```python
from build123d import *

# Parameters (mm, degrees)
SKETCH1_W                  = 15
SKETCH1_H                  = 20
BOSS_EXTRUDE1_DEPTH        = 10
F_4_2_4_2_DIAMETER_HOLE1_D = 4.2
SKETCH4_W                  = 10
SKETCH4_H                  = 20
BOSS_EXTRUDE2_DEPTH        = 15
SKETCH5_W                  = 15
SKETCH5_H                  = 20
BOSS_EXTRUDE3_DEPTH        = 20
CHAMFER1_SIZE              = 10
CHAMFER2_SIZE              = 15
SKETCH6_W                  = 5
SKETCH6_H                  = 20
CUT_EXTRUDE1_DEPTH         = 10
SKETCH8_W                  = 15
SKETCH8_H                  = 20
BOSS_EXTRUDE4_DEPTH        = 10
CHAMFER3_SIZE              = 10
SKETCH7_W                  = 10
SKETCH7_H                  = 20
BOSS_EXTRUDE5_DEPTH        = 25
FILLET5_R                  = 3.175
SKETCH9_W                  = 10
SKETCH9_H                  = 10
CUT_EXTRUDE4_DEPTH         = 37
SKETCH15_W                 = 35.287710309
SKETCH15_H                 = 35.27052657
CUT_EXTRUDE5_DEPTH         = 10
SKETCH16_W                 = 32
SKETCH16_H                 = 10
CUT_EXTRUDE6_DEPTH         = 46
MOVE_FACE1_BY              = 5
SKETCH19_W                 = 2
SKETCH19_H                 = 6.2
BOSS_EXTRUDE6_DEPTH        = 2
FILLET6_R                  = 6.35
FILLET7_R                  = 3.175


# Some blends are built 0.0001 mm under size
with BuildPart() as part:
    # Sketch1 → Boss-Extrude1 (new body)
    with BuildSketch(Plane.XY):
        with Locations((7.5, 10)):
            Rectangle(SKETCH1_W, SKETCH1_H)
    extrude(amount=BOSS_EXTRUDE1_DEPTH)

    # Ø4.2 (4.2) Diameter Hole1 (through all)
    with Locations(Plane.XY.offset(10)):
        with Locations((8, 17)):
            Hole(F_4_2_4_2_DIAMETER_HOLE1_D / 2)

    # Sketch4 → Boss-Extrude2 (add)
    with BuildSketch(Plane(origin=(15, 0, 0), x_dir=(0, 0, -1), z_dir=(1, 0, 0))):
        with Locations((-5, 10)):
            Rectangle(SKETCH4_W, SKETCH4_H)
    extrude(amount=BOSS_EXTRUDE2_DEPTH)

    # Sketch5 → Boss-Extrude3 (add)
    with BuildSketch(Plane(origin=(0, 0, 0), x_dir=(-1, 0, 0), z_dir=(0, 0, -1))):
        with Locations((-22.5, 10)):
            Rectangle(SKETCH5_W, SKETCH5_H)
    extrude(amount=BOSS_EXTRUDE3_DEPTH)

    # Chamfer1
    # the kernel refuses this chamfer: 10 mm, written as the material it adds along each edge
    with BuildSketch(Plane(origin=(15, 20, 0), x_dir=(-0.9996219169112968, 0, 0.027495876610586372), z_dir=(0, -1, 0))) as chamfer1_piece_1_section:
        Polygon((CHAMFER1_SIZE * 0.999621916911, CHAMFER1_SIZE * 0.0274958766106), (-CHAMFER1_SIZE * 0.0274958766106, CHAMFER1_SIZE * 0.999621916911), (0, 0), align=None)
    chamfer1_piece_1 = extrude(amount=20, mode=Mode.PRIVATE)
    chamfer1_piece_1 = chamfer1_piece_1 - Plane(origin=(8, 17, -3.373966189), x_dir=(-1, 0, 0), z_dir=(0, 0, -1)) * Cylinder(2.1, 80, mode=Mode.PRIVATE)
    add(chamfer1_piece_1)

    # Chamfer2
    chamfer2_edges = [part.edges().sort_by_distance(p)[0] for p in [
        (30, 10, 10),
    ]]
    chamfer(chamfer2_edges, length=CHAMFER2_SIZE)

    # Sketch6 → Cut-Extrude1 (cut)
    with BuildSketch(Plane(origin=(0, 0, 0), x_dir=(-1, 0, 0), z_dir=(0, 0, -1))):
        with Locations((-2.5, 10)):
            Rectangle(SKETCH6_W, SKETCH6_H)
    extrude(amount=-CUT_EXTRUDE1_DEPTH, mode=Mode.SUBTRACT)

    # Sketch8 → Boss-Extrude4 (add)
    with BuildSketch(Plane(origin=(30, 0, 0), x_dir=(0, 0, -1), z_dir=(1, 0, 0))):
        with Locations((12.5, 10)):
            Rectangle(SKETCH8_W, SKETCH8_H)
    extrude(amount=BOSS_EXTRUDE4_DEPTH)

    # Chamfer3
    chamfer3_edges = [part.edges().sort_by_distance(p)[0] for p in [
        (40, 10, -5),
    ]]
    chamfer(chamfer3_edges, length=CHAMFER3_SIZE - 0.0001)  # a hair under: the kernel refuses the full size

    # Sketch7 → Boss-Extrude5 (add)
    with BuildSketch(Plane(origin=(30, 0, 0), x_dir=(0, 0, -1), z_dir=(1, 0, 0))):
        with Locations((15, 10)):
            Rectangle(SKETCH7_W, SKETCH7_H)
    extrude(amount=BOSS_EXTRUDE5_DEPTH)

    # Fillet5
    fillet5_edges = [part.edges().sort_by_distance(p)[0] for p in [
        (35.0001, 10, -10),
    ]]
    fillet(fillet5_edges, radius=FILLET5_R)

    # Sketch9 → Cut-Extrude4 (cut)
    with BuildSketch(Plane(origin=(0, 0, -20), x_dir=(-1, 0, 0), z_dir=(0, 0, -1))):
        with Locations((-10, 5)):
            Rectangle(SKETCH9_W, SKETCH9_H)
    extrude(amount=-CUT_EXTRUDE4_DEPTH, mode=Mode.SUBTRACT)

    # Sketch14 → CBORE for M5 SBHCS2 (revolve, cut)
    with BuildSketch(Plane(origin=(45, 10, 10), x_dir=(0, -1, 0), z_dir=(1, 0, 0))):
        Polygon((0, 0), (0, 30), (2.65, 30), (2.65, 22.75), (5.25, 22.75), (5.25, 0.020977491), (5.275, 0), align=None)
    revolve(axis=Axis((45, 10, 16.35), (0, 0, -1)), mode=Mode.SUBTRACT)

    # Sketch15 → Cut-Extrude5 (cut)
    with BuildSketch(Plane(origin=(2.5, 0, 2.5), x_dir=(-0.707106781186544, 0, 0.7071067811865511), z_dir=(-0.7071067811865511, 0, -0.707106781186544))):
        with Locations((-14.684853065, 9.385409348)):
            Rectangle(SKETCH15_W, SKETCH15_H)
    extrude(amount=CUT_EXTRUDE5_DEPTH, mode=Mode.SUBTRACT)

    # Sketch16 → Cut-Extrude6 (cut)
    with BuildSketch(Plane(origin=(0, 0, -20), x_dir=(-1, 0, 0), z_dir=(0, 0, -1))):
        with Locations((-21, 5)):
            Rectangle(SKETCH16_W, SKETCH16_H)
    extrude(amount=-CUT_EXTRUDE6_DEPTH, mode=Mode.SUBTRACT)

    # Move Face1: a face moved outward by 5.0
    extrude(part.faces().sort_by_distance((55, 10, -15))[0], amount=MOVE_FACE1_BY, dir=(1, 0, 0))

    # Sketch19 → Boss-Extrude6 (add)
    with BuildSketch(Plane(origin=(0, 0, -20), x_dir=(-1, 0, 0), z_dir=(0, 0, -1))):
        with Locations((-59, 10)):
            Rectangle(SKETCH19_W, SKETCH19_H)
    extrude(amount=BOSS_EXTRUDE6_DEPTH)

    # Fillet6
    # the kernel refuses this fillet: 6.35 mm, written as the material it adds along each edge
    with BuildSketch(Plane(origin=(58, 13.1, -20), x_dir=(-1, 0, 0), z_dir=(0, -1, 0))) as fillet6_piece_1:
        with BuildLine():
            CenterArc((4.626013402, 6.35), FILLET6_R, 223.238703461, 46.761296539)
            Line((0, 2), (-0.092520268, 1.913))
            ThreePointArc((-0.092520268, 1.913), (-0.127, 1), (-0.127, 0))
            Line((-0.127, 0), (0, -0.127))
            Line((0, -0.127), (4.626013402, -0.127))
            Line((4.626013402, -0.127), (4.626013402, 0))
        make_face()
    extrude(amount=6.2)

    # Fillet7
    fillet7_edges = [part.edges().sort_by_distance(p)[0] for p in [
        (37, 10, -15),
    ]]
    fillet(fillet7_edges, radius=FILLET7_R)


solid = part.part
```
Could you check a few things on this model? Use its own coordinates, in mm. A direction names the side the tool comes from. Coordinates: 2 decimals unless noted, no trailing zeros. Loops run counter-clockwise (first coordinate to the right, second up) from the corner with the lowest first, then second, coordinate; pieces in that order, holes last.
1) Will these pins go through, and if not, where does the flat tip stop? pin 1 Ø3 at (x, y) = (43, 11.5) entering from +Z; pin 2 Ø6.5 at (x, y) = (8, 17) entering from -Z; pin 3 Ø3 at (x, y) = (53, 10.5) entering from +Z.
Reported:
pin 1: stops at z = -12.75
pin 2: stops at z = -6.25
pin 3: stops at z = -10
2) Imagine slicing it at D-D (x = 8). List the corners of the cut face in (y, z) for me, and give its area (3 significant figures).
Reported:
outline: (10, -3) - (14.9, -3) - (14.9, 10) - (10, 10) - close; (19.1, -3) - (20, -3) - (20, 10) - (19.1, 10) - close
area: 75.4 mm2
3) Thinking about a two-plate mould opening in X: for faces 1 (the face through (58, 13.1, -21)), 2 (the face through (47, 12, -12.75)), 3 (the face through (55.927, 10.043, -20.536)), which applies, released by +X, released by -X, zero draft, split by the parting line, or undercut?
Reported:
face 1: zero draft
face 2: undercut
face 3: released by -X
4) Which directions (+Z, -Z, +X, -X, +Y, -Y) give clear straight access to the entire face, cutting with the end or side of a thin tool? Please do faces 4 (the face through (39.795, 10.683, -11.356)), 5 (the face through (20, 10, -5)), 6 (the face through (58, 6.9, -21)), 7 (the face through (51, 10, -10)).
Reported:
face 4: +Z
face 5: +Z, -Z, -X, -Y
face 6: -Z, +X, -X, -Y
face 7: +Z, +X, +Y, -Y
5) Imagine slicing it at C-C (z = 8). List the corners of the cut face in (x, y) for me.
Reported:
outline: (5, 10) - (17, 10) - (17, 20) - (5, 20) - close; hole circle Ø4.2 at (8, 17)
6) Imagine slicing it at A-A (x = 45). List the corners of the cut face in (y, z) for me.
Reported:
outline: (0, -20) - (7.35, -20) - (7.35, -12.75) - (4.75, -12.75) - (4.75, -10) - (0, -10) - close; (12.65, -20) - (20, -20) - (20, -10) - (15.25, -10) - (15.25, -12.75) - (12.65, -12.75) - close
7) Please list where these lines run through material, in increasing order: line 1 along Y through (x, z) = (45, -11.95); line 2 along Y through (x, z) = (8, -1); line 3 along X through (y, z) = (10.25, -16.5).
Reported:
line 1: y = 0 to 4.75, 15.25 to 20
line 2: y = 10 to 14.9, 19.1 to 20
line 3: x = 21.5 to 42.36, 47.64 to 60
